Drawing for the job (mm, zero at the part's lowest x, y, z). A direction names the side the tool comes from. Give positions to 0.01 mm unless a question says otherwise; leave off trailing zeros. Order: outer loops, then holes, each group sorted by start corner. A loop starts at its lowest first (then second) coordinate and runs counter-clockwise, first axis right, second up. Notation, with made-up numbers: (56, -26) - (74, -26) arc R18 cw to (74, -4) - close; hole circle Ø11 at (46.25, 0.5). An arc over 180 degrees is marked (long way). One line per item, written item: value.
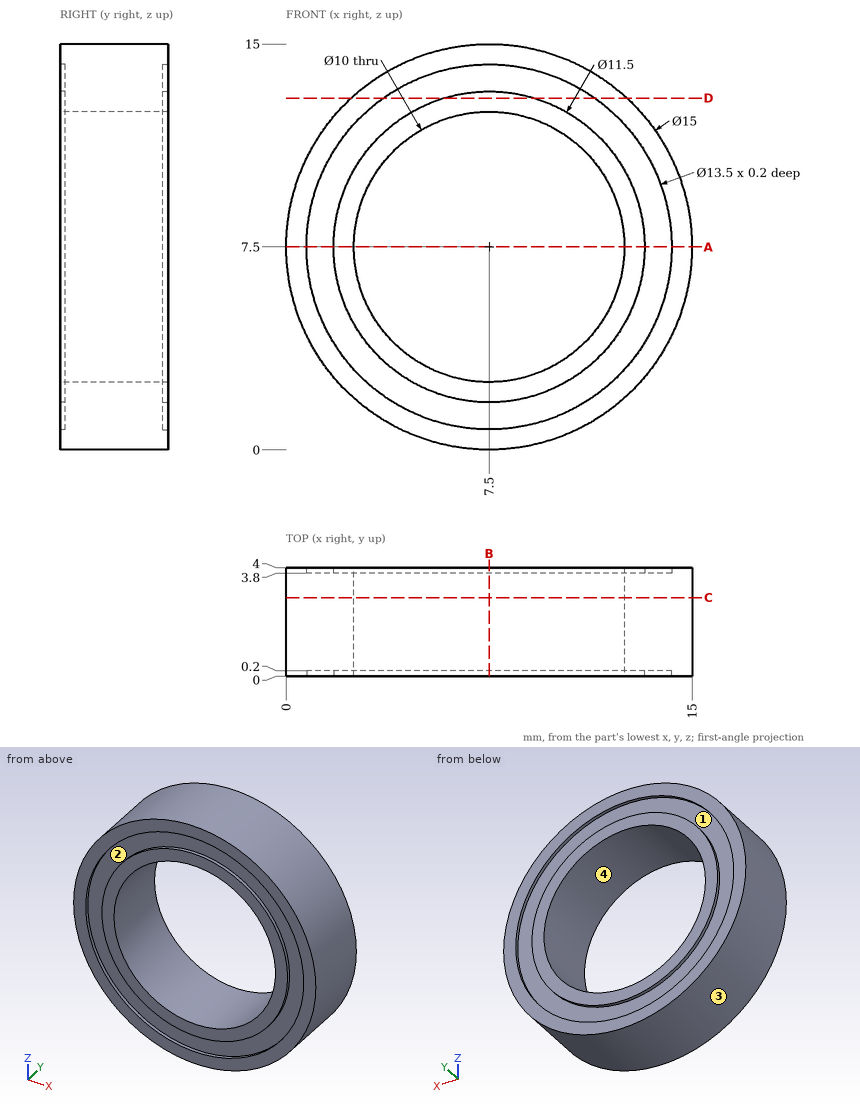
1) Cut at A-A, the plane z = 7.5. Give the cut face in (x, y).
Outcome:
outline: (0, 0) - (0.75, 0) - (0.75, 0.2) - (1.75, 0.2) - (1.75, 0) - (2.5, 0) - (2.5, 4) - (1.75, 4) - (1.75, 3.8) - (0.75, 3.8) - (0.75, 4) - (0, 4) - close; (12.5, 0) - (13.25, 0) - (13.25, 0.2) - (14.25, 0.2) - (14.25, 0) - (15, 0) - (15, 4) - (14.25, 4) - (14.25, 3.8) - (13.25, 3.8) - (13.25, 4) - (12.5, 4) - close
2) Drill centre lines: line 1 along Z through (x, y) = (7.5, 3.95); line 2 along Z through (x, y) = (6, 2.4); line 3 along X through (y, z) = (3.6, 3.25). Where is each one in solid material? Low to high. Write a range as from..to.
Outcome:
line 1: z = 0..0.75, 1.75..2.5, 12.5..13.25, 14.25..15
line 2: z = 0.15..2.73, 12.27..14.85
line 3: x = 1.32..4.87, 10.13..13.68
3) Mould opens along X. For the marked faces 3 and 4 say: released by +X, released by -X, zero draft, split by the parting line, or undercut.
Outcome:
face 3: split by the parting line
face 4: undercut
4) Cut at C-C, the plane y = 2.9. Give the cut face in (x, z), then the cut area to 3 significant figures.
Outcome:
outline: circle Ø15 at (7.5, 7.5); hole circle Ø10 at (7.5, 7.5)
area: 98.2 mm^2
5) Cut at B-B, the plane x = 7.5. Give the cut face in (y, z), then the cut area to 3 significant figures.
Outcome:
outline: (0, 0) - (4, 0) - (4, 0.75) - (3.8, 0.75) - (3.8, 1.75) - (4, 1.75) - (4, 2.5) - (0, 2.5) - (0, 1.75) - (0.2, 1.75) - (0.2, 0.75) - (0, 0.75) - close; (0, 12.5) - (4, 12.5) - (4, 13.25) - (3.8, 13.25) - (3.8, 14.25) - (4, 14.25) - (4, 15) - (0, 15) - (0, 14.25) - (0.2, 14.25) - (0.2, 13.25) - (0, 13.25) - close
area: 19.2 mm^2
6) Cut at D-D, the plane z = 13. Give the cut face in (x, y).
Outcome:
outline: (2.4, 0) - (3.59, 0) - (3.59, 0.2) - (5.82, 0.2) - (5.82, 0) - (9.18, 0) - (9.18, 0.2) - (11.41, 0.2) - (11.41, 0) - (12.6, 0) - (12.6, 4) - (11.41, 4) - (11.41, 3.8) - (9.18, 3.8) - (9.18, 4) - (5.82, 4) - (5.82, 3.8) - (3.59, 3.8) - (3.59, 4) - (2.4, 4) - close
7) Pin check, flat tips, straight feed: pin 1 (6 mm diameter, centred on x = 7.5, z = 7.5, fed in from -Y); pin 2 (1 mm diameter, centred on x = 10, y = 2, fed in from -Z); pin 3 (2 mm diameter, centred on y = 3.5, z = 6, fed in from +X). Stop position of each tip, or through.
Outcome:
pin 1: passes through
pin 2: stops at z = 0.27
pin 3: stops at x = 14.98
8) Which spindle directions (+Z, -Z, +X, -X, +Y, -Y) get a long thin tool onto all of the face, cutting with end or side? Do the marked faces 1 and 2. Say none if no direction does.
Outcome:
face 1: +Y
face 2: -Y
